from build123d import *

# Parameters (mm, degrees)
F1_DEPTH = 10
F2_R     = 1
F3_W     = 4.5
F3_H     = 4.5
F4_DEPTH = 4.5


with BuildPart() as f1:
    # F0 (on Front) → F1 (new body)
    with BuildSketch(Plane.XZ):
        Polygon((10.715883, -20.351163), (0, 0), (-8.806125, 0), (16.310085, -48.875057), (16.310085, -19.975057), (10.715883, -8.351163), align=None)
    extrude(amount=F1_DEPTH)

    # F2
    f2_edges = [f1.edges().sort_by_distance(p)[0] for p in [
        (13.512984, -10, -14.16311),
        (3.75198, -10, -24.437528),
        (5.357942, -10, -10.175582),
        (10.715883, -10, -14.351163),
        (16.310085, -10, -34.425057),
        (-4.403063, -10, 0),
    ]]
    fillet(f2_edges, radius=F2_R)

    # F3 (on face) → F4 (join)
    with BuildSketch(Plane.XY):
        with Locations((-5.718835, -3.562355)):
            Rectangle(F3_W, F3_H)
    extrude(amount=F4_DEPTH)


solid = f1.part
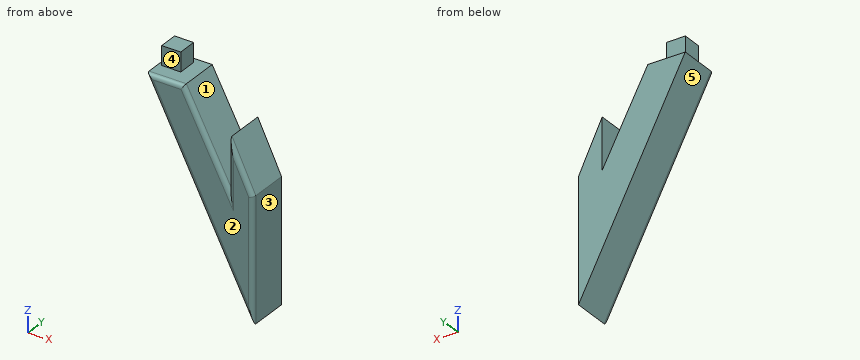
Part model, mm, in its own coordinate system. Face numbers are marked on the shaded views. A direction names the side the tool comes from. Coordinates: 2 decimals unless noted, no trailing zeros. Order: outer loops, then holes, each group sorted by start corner. A loop starts at its lowest first (then second) coordinate and runs counter-clockwise, first axis right, second up. Notation, with made-up numbers: M 13,24 L 61,24 A24 cw 61,62 Z; hole C 12,-23 d4. An arc over 180 degrees is marked long. Use a Markdown table: item, result.
(1) Cut at A-A on y = -5.25. Write the cut outline in (x, z), then the cut area to 3 significant figures.
A:
| item | result |
|---|---|
| outline | M -8.81,0 L 16.31,-48.88 L 16.31,-19.98 L 10.72,-8.35 L 10.72,-20.35 L 0,0 L -3.47,0 L -3.47,4.5 L -7.97,4.5 L -7.97,0 Z |
| area | 446 mm^2 |
(2) Tool access for the marked faces 4 and 5: list every direction of +Z, -Z, +X, -X, +Y, -Y with a clear straight run to the whole face (end or side of a thin tool).
A:
| item | result |
|---|---|
| face 4 | +Z, +X, -X, -Y |
| face 5 | -Z, -X, +Y, -Y |
(3) Pull direction X, two halves, no side cores. Call the marked faces 1, 2 and 3: released by +X, released by -X, zero draft, split by the parting line, or undercut.
A:
| item | result |
|---|---|
| face 1 | undercut |
| face 2 | zero draft |
| face 3 | released by +X |
(4) Cut at C-C on y = -8. Write the cut outline in (x, z).
A:
| item | result |
|---|---|
| outline | M -8.81,0 L 16.31,-48.88 L 16.31,-19.98 L 10.72,-8.35 L 10.72,-20.35 L 0,0 Z |
(5) Flat gauge pins, fed straight in: pin 1 (3.5 mm diameter, centred on x = -5, z = 2, fed in from +Y); pin 2 (6 mm diameter, centred on x = -5, y = -8.5, fed in from -Z); pin 3 (3.5 mm diameter, centred on y = -4, z = 2.5, fed in from -X). Where does each tip first touch, or does it go through?
A:
| item | result |
|---|---|
| pin 1 | stops at y = -1.31 |
| pin 2 | stops at z = -13.24 |
| pin 3 | stops at x = -7.97 |
(6) Cut at B-B on z = 0.5. Write the cut outline in (x, y).
A:
| item | result |
|---|---|
| outline | M -7.97,-5.81 L -3.47,-5.81 L -3.47,-1.31 L -7.97,-1.31 Z |
(7) Probe L1, parallel to X at y = -0.75, z = -29; L2, parallel to Z at x = 3.75, y = -2.5; L3, parallel to X at y = -7.5, z = -1.5. List the from-to ranges inside material, lowest first.
A:
| item | result |
|---|---|
| L1 | x = 6.1 to 16.31 |
| L2 | z = -24.43 to -7.12 |
| L3 | x = -8.04 to 0.79 |
